```python
from build123d import *

# Parameters (mm, degrees)
SKETCH2_W           = 152.4
SKETCH2_H           = 120.65
BOSS_EXTRUDE2_DEPTH = 12.7
SKETCH4_W           = 50.8
SKETCH4_H           = 25.4
BOSS_EXTRUDE3_DEPTH = 95.25
CUT_EXTRUDE1_DEPTH  = 179.930335606


with BuildPart() as part:
    # Sketch2 → Boss-Extrude2 (new body)
    with BuildSketch(Plane(origin=(0, 0, 0), x_dir=(1, 0, 0), z_dir=(0, 1, 0))):
        Rectangle(SKETCH2_W, SKETCH2_H)
    extrude(amount=BOSS_EXTRUDE2_DEPTH)

    # Sketch4 → Boss-Extrude3 (add)
    with BuildSketch(Plane(origin=(0, 12.7, 0), x_dir=(1, 0, 0), z_dir=(0, 1, 0))):
        with Locations((0, -47.625)):
            Rectangle(SKETCH4_W, SKETCH4_H)
    boss_extrude3 = extrude(amount=BOSS_EXTRUDE3_DEPTH)

    # Mirror1: Boss-Extrude3 across plane
    add(boss_extrude3.mirror(Plane.XY))

    # Sketch6 → Cut-Extrude1 (cut, through all)
    with BuildSketch(Plane.XY.offset(60.325)):
        with BuildLine():
            Line((-6.911847883, 107.95), (5.788152117, 107.95))
            Line((5.788152117, 107.95), (5.788152117, 82.912540003))
            ThreePointArc((5.788152117, 82.912540003), (0.627347046, 55.576279674), (-6.911847883, 82.354359843))
            Line((-6.911847883, 82.354359843), (-6.911847883, 107.95))
        make_face()
    extrude(amount=-CUT_EXTRUDE1_DEPTH, mode=Mode.SUBTRACT)


solid = part.part
```
CAD build for the part. Positions are in the model's coordinates, mm. A direction names the side the tool comes from. Round coordinates to 2 decimals unless told otherwise and drop trailing zeros. Order: outer loops, then holes, each group sorted by start corner. A loop starts at its lowest first (then second) coordinate and runs counter-clockwise, first axis right, second up. Notation, with made-up numbers: (84.5, 73) - (108.5, 73) arc R17 ccw to (108.5, 101) - close; hole circle Ø4 at (23, -18.5). An arc over 180 degrees is marked (long way). Answer as CSV lines item,"result". Start each with the question number.
1. Saw through at D-D, the plane y = 92. Write the cut outline in (x, z) (3 decimals).
2. Pin check, flat tips, straight feed: pin 1 (7.5 mm diameter, centred on y = 79, z = 50.5, fed in from +X); pin 2 (3 mm diameter, centred on x = 55, z = -4.5, fed in from +Y); pin 3 (12 mm diameter, centred on y = 87.5, z = -28.5, fed in from +X); pin 4 (20.5 mm diameter, centred on y = 55.5, z = -52, fed in from -X). Stop position of each tip, or through.
3. Saw through at A-A, the plane y = 46.5. Write the cut outline in (x, z) (3 decimals).
4. Drill centre lines: L1, parallel to X at y = 69, z = -43; L2, parallel to Y at x = -19.5, z = 12.5; L3, parallel to Y at x = 0, z = -52.5. Where is each one in solid material? Low to high. Write a range as [from, to].
5. Saw through at C-C, the plane x = 0. Write the cut outline in (y, z) (1 decimal), and give its area (3 significant figures).
6. Pull direction X, two halves, no side cores. Call faces 6 (the face through (-25.4, 60, -48)), 7 (the face through (-6.912, 95, -47)), 8 (the face through (0, 34, -60.325)): +X half, -X half, draft (parallel to the pull), parting line (faces both ways), or undercut.
7. Tool access for faces 1 (the face through (5.788, 96, 48)), 2 (the face through (-76.2, 6, 1)), 3 (the face through (25.4, 60, 48)), 4 (the face through (0, 49, -34.925)), 5 (the face through (1.16, 55.61, -47.45)): list every direction of +Z, -Z, +X, -X, +Y, -Y with a clear straight run to the whole face (end or side of a thin tool).
8. Saw through at B-B, the plane y = 69.85. Write the cut outline in (x, z) (1 decimal), and give its area (3 significant figures).
Model answer:
1,outline,"(-25.4, -60.325) - (-6.912, -60.325) - (-6.912, -34.925) - (-25.4, -34.925) - close; (-25.4, 34.925) - (-6.912, 34.925) - (-6.912, 60.325) - (-25.4, 60.325) - close; (5.788, -60.325) - (25.4, -60.325) - (25.4, -34.925) - (5.788, -34.925) - close; (5.788, 34.925) - (25.4, 34.925) - (25.4, 60.325) - (5.788, 60.325) - close"
2,pin 1,"stops at x = 25.4"
2,pin 2,"stops at y = 12.7"
2,pin 3,"passes through"
2,pin 4,"stops at x = -25.4"
3,outline,"(-25.4, -60.325) - (25.4, -60.325) - (25.4, -34.925) - (-25.4, -34.925) - close; (-25.4, 34.925) - (25.4, 34.925) - (25.4, 60.325) - (-25.4, 60.325) - close"
4,L1,"x = [-25.4, -14.26], [14.26, 25.4]"
4,L2,"y = [0, 12.7]"
4,L3,"y = [0, 55.56]"
5,outline,"(0, -60.3) - (55.6, -60.3) - (55.6, -34.9) - (12.7, -34.9) - (12.7, 34.9) - (55.6, 34.9) - (55.6, 60.3) - (0, 60.3) - close"
5,area,"3,710 mm²"
6,face 6,"-X half"
6,face 7,"undercut"
6,face 8,"draft"
7,face 1,"+Z, -Z, +Y"
7,face 2,"+Z, -Z, -X, +Y, -Y"
7,face 3,"+Z, -Z, +X, +Y"
7,face 4,"+X, -X, +Y"
7,face 5,"+Z, -Z"
8,outline,"(-25.4, -60.3) - (-14.3, -60.3) - (-14.3, -34.9) - (-25.4, -34.9) - close; (-25.4, 34.9) - (-14.3, 34.9) - (-14.3, 60.3) - (-25.4, 60.3) - close; (14.3, -60.3) - (25.4, -60.3) - (25.4, -34.9) - (14.3, -34.9) - close; (14.3, 34.9) - (25.4, 34.9) - (25.4, 60.3) - (14.3, 60.3) - close"
8,area,"1,130 mm²"
